```python
from build123d import *

# Parameters (mm, degrees)
SKETCH1_W                    = 52.8
SKETCH1_H                    = 30.6
EXT_BODY_DEPTH               = 13.8
AUTO_SWITCH_MOUNTING_DEPTH   = 57.677773421
SKETCH3_R                    = 8.5
CYL_BORE_DEPTH               = 2
M4X0_7_TAPPED_HOLE1_D        = 3.3
M4X0_7_TAPPED_HOLE1_DEPTH    = 10.1
M4X0_7_TAPPED_HOLE1_TIP      = 0.991420021
F_3_0_3_DIAMETER_HOLE1_D     = 3
F_3_0_3_DIAMETER_HOLE1_DEPTH = 3
F_3_0_3_DIAMETER_HOLE1_TIP   = 0.901290929
M4X0_7_TAPPED_HOLE2_D        = 3.3
M4X0_7_TAPPED_HOLE2_DEPTH    = 10.1
M4X0_7_TAPPED_HOLE2_TIP      = 0.991420021
M4X0_7_TAPPED_HOLE3_D        = 3.3
M4X0_7_TAPPED_HOLE3_DEPTH    = 10.1
M4X0_7_TAPPED_HOLE3_TIP      = 0.991420021
M4X0_7_TAPPED_HOLE4_D        = 3.3
M4X0_7_TAPPED_HOLE4_DEPTH    = 6.6
M4X0_7_TAPPED_HOLE4_TIP      = 0.991420021
M5X0_8_TAPPED_HOLE1_D        = 4.2
M5X0_8_TAPPED_HOLE1_DEPTH    = 6
M5X0_8_TAPPED_HOLE1_TIP      = 1.2618073
BOSS_EXTRUDE2_DEPTH          = 19
CHAMFER1_SIZE                = 0.25


with BuildPart() as part:
    # Sketch1 → EXT BODY (new, symmetric)
    with BuildSketch(Plane.XY):
        Rectangle(SKETCH1_W, SKETCH1_H)
    extrude(amount=EXT_BODY_DEPTH, both=True)

    # Sketch2 → AUTO SWITCH MOUNTING (cut, through all)
    with BuildSketch(Plane(origin=(26.4, 0, 0), x_dir=(0, 0, -1), z_dir=(1, 0, 0))):
        Polygon((2.5, 15.3), (-2.5, 15.3), (-2.5, 13.6), (-3.1, 13), (-3.1, 9.5), (3.1, 9.5), (3.1, 13), (2.5, 13.6), align=None)
        with BuildLine():
            Line((-13.022875656, 7.3), (-13.8, 7.3))
            Line((-13.8, 7.3), (-13.8, 4.3))
            Line((-13.8, 4.3), (-13.022875656, 4.3))
            ThreePointArc((-13.022875656, 4.3), (-9.7, 5.8), (-13.022875656, 7.3))
        make_face()
        with BuildLine():
            Line((-13.8, -7.3), (-13.8, -4.3))
            Line((-13.8, -4.3), (-13.022875656, -4.3))
            ThreePointArc((-13.022875656, -4.3), (-9.7, -5.8), (-13.022875656, -7.3))
            Line((-13.022875656, -7.3), (-13.8, -7.3))
        make_face()
        Polygon((-3.1, -9.5), (3.1, -9.5), (3.1, -13), (2.5, -13.6), (2.5, -15.3), (-2.5, -15.3), (-2.5, -13.6), (-3.1, -13), align=None)
        with BuildLine():
            Line((13.022875656, -7.3), (13.8, -7.3))
            Line((13.8, -7.3), (13.8, -4.3))
            Line((13.8, -4.3), (13.022875656, -4.3))
            ThreePointArc((13.022875656, -4.3), (9.7, -5.8), (13.022875656, -7.3))
        make_face()
        with BuildLine():
            Line((13.8, 7.3), (13.8, 4.3))
            Line((13.8, 4.3), (13.022875656, 4.3))
            ThreePointArc((13.022875656, 4.3), (9.7, 5.8), (13.022875656, 7.3))
            Line((13.022875656, 7.3), (13.8, 7.3))
        make_face()
    extrude(amount=-AUTO_SWITCH_MOUNTING_DEPTH, mode=Mode.SUBTRACT)

    # Sketch3 → CYL BORE (cut)
    with BuildSketch(Plane(origin=(26.4, 0, 0), x_dir=(0, 0, -1), z_dir=(1, 0, 0))):
        Circle(SKETCH3_R)
    extrude(amount=-CYL_BORE_DEPTH, mode=Mode.SUBTRACT)

    # M4x0.7 Tapped Hole1
    with Locations(Plane(origin=(26.4, 0, 0), x_dir=(0, 0, -1), z_dir=(1, 0, 0))):
        with Locations((-7.5, -11), (7.5, 11)):
            Hole(M4X0_7_TAPPED_HOLE1_D / 2, depth=M4X0_7_TAPPED_HOLE1_DEPTH)
            with Locations((0, 0, -(M4X0_7_TAPPED_HOLE1_DEPTH + M4X0_7_TAPPED_HOLE1_TIP / 2))):  # 118° drill point
                Cone(0, M4X0_7_TAPPED_HOLE1_D / 2, M4X0_7_TAPPED_HOLE1_TIP, mode=Mode.SUBTRACT)

    # Ø3.0 (3) Diameter Hole1
    with Locations(Plane(origin=(26.4, 0, 0), x_dir=(0, 0, -1), z_dir=(1, 0, 0))):
        with Locations((-6.5, 11)):
            Hole(F_3_0_3_DIAMETER_HOLE1_D / 2, depth=F_3_0_3_DIAMETER_HOLE1_DEPTH)
            with Locations((0, 0, -(F_3_0_3_DIAMETER_HOLE1_DEPTH + F_3_0_3_DIAMETER_HOLE1_TIP / 2))):  # 118° drill point
                Cone(0, F_3_0_3_DIAMETER_HOLE1_D / 2, F_3_0_3_DIAMETER_HOLE1_TIP, mode=Mode.SUBTRACT)

    # M4x0.7 Tapped Hole2
    with Locations(Plane.XY.offset(13.8)):
        with Locations((1.9, 12), (1.9, -12)):
            Hole(M4X0_7_TAPPED_HOLE2_D / 2, depth=M4X0_7_TAPPED_HOLE2_DEPTH)
            with Locations((0, 0, -(M4X0_7_TAPPED_HOLE2_DEPTH + M4X0_7_TAPPED_HOLE2_TIP / 2))):  # 118° drill point
                Cone(0, M4X0_7_TAPPED_HOLE2_D / 2, M4X0_7_TAPPED_HOLE2_TIP, mode=Mode.SUBTRACT)

    # M4x0.7 Tapped Hole3
    with Locations(Plane(origin=(0, 0, -13.8), x_dir=(-1, 0, 0), z_dir=(0, 0, -1))):
        with Locations((-1.9, 12), (-1.9, -12)):
            Hole(M4X0_7_TAPPED_HOLE3_D / 2, depth=M4X0_7_TAPPED_HOLE3_DEPTH)
            with Locations((0, 0, -(M4X0_7_TAPPED_HOLE3_DEPTH + M4X0_7_TAPPED_HOLE3_TIP / 2))):  # 118° drill point
                Cone(0, M4X0_7_TAPPED_HOLE3_D / 2, M4X0_7_TAPPED_HOLE3_TIP, mode=Mode.SUBTRACT)

    # M4x0.7 Tapped Hole4
    with Locations(Plane(origin=(0, 15.3, 0), x_dir=(1, 0, 0), z_dir=(0, 1, 0))):
        with Locations((-3.6, 8), (-3.6, -8)):
            Hole(M4X0_7_TAPPED_HOLE4_D / 2, depth=M4X0_7_TAPPED_HOLE4_DEPTH)
            with Locations((0, 0, -(M4X0_7_TAPPED_HOLE4_DEPTH + M4X0_7_TAPPED_HOLE4_TIP / 2))):  # 118° drill point
                Cone(0, M4X0_7_TAPPED_HOLE4_D / 2, M4X0_7_TAPPED_HOLE4_TIP, mode=Mode.SUBTRACT)

    # M5x0.8 Tapped Hole1
    with Locations(Plane(origin=(0, -15.3, 0), x_dir=(-1, 0, 0), z_dir=(0, -1, 0))):
        with Locations((-7.4, -7.5), (-18.9, 7.5)):
            Hole(M5X0_8_TAPPED_HOLE1_D / 2, depth=M5X0_8_TAPPED_HOLE1_DEPTH)
            with Locations((0, 0, -(M5X0_8_TAPPED_HOLE1_DEPTH + M5X0_8_TAPPED_HOLE1_TIP / 2))):  # 118° drill point
                Cone(0, M5X0_8_TAPPED_HOLE1_D / 2, M5X0_8_TAPPED_HOLE1_TIP, mode=Mode.SUBTRACT)

    # Sketch21 → Boss-Extrude2 (add, symmetric)
    with BuildSketch(Plane(origin=(0, 0, 0), x_dir=(1, 0, 0), z_dir=(0, 1, 0))):
        with BuildLine():
            Line((-33.9, 4.5), (-33.9, 11.25))
            Line((-33.9, 11.25), (-26.4, 11.25))
            Line((-26.4, 11.25), (-26.4, -11.25))
            Line((-26.4, -11.25), (-33.9, -11.25))
            Line((-33.9, -11.25), (-33.9, -4.5))
            Line((-33.9, -4.5), (-33.025, -4.5))
            ThreePointArc((-33.025, -4.5), (-32.025, -5.5), (-31.025, -4.5))
            Line((-31.025, -4.5), (-30.15, -4.5))
            Line((-30.15, -4.5), (-30.15, 4.5))
            Line((-30.15, 4.5), (-31.025, 4.5))
            ThreePointArc((-31.025, 4.5), (-32.025, 5.5), (-33.025, 4.5))
            Line((-33.025, 4.5), (-33.9, 4.5))
        make_face()
    extrude(amount=BOSS_EXTRUDE2_DEPTH, both=True)

    # Chamfer1
    chamfer1_edges = [part.edges().sort_by_distance(p)[0] for p in [
        (-33.9, 0, -4.5),
        (-33.9, 0, 4.5),
    ]]
    chamfer(chamfer1_edges, length=CHAMFER1_SIZE)


solid = part.part
```
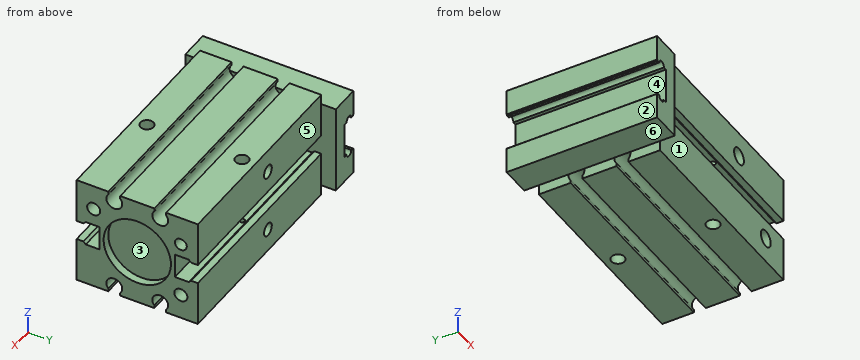
Geometry: final body of the model. Coordinates: model frame, mm. Face numbers are marked on the shaded views. A direction names the side the tool comes from. Round coordinates to 2 decimals unless told otherwise and drop trailing zeros. Write each loop counter-clockwise with the first axis right and the second up, starting at its lowest first coordinate (ties: lowest second). Pieces come first, ordered by that corner, then holes.
Item 1: Section query A-A (z = 0.25). Return loops of the section in (x, y), plus the area to 3 significant figures.
Item 2: Section query D-D (y = 5.5). Return loops of the section in (x, z) (3 decimals), plus the area to 3 significant figures.
Item 3: Mould query, pull axis Y, two halves, no side actions, for the marked faces 1, 2 and 3. Classes: +Y half, -Y half, draft (parallel to the pull), parting line (faces both ways), or undercut.
Item 4: Pin query (flat end, axial travel): P1, Ø0.5, axis at x = -33.5, y = 0.5, coming from the +Z side; P2, Ø12, axis at x = -12, z = 10.5, coming from the -Y side; P3, Ø3, axis at x = 1.9, y = -12, coming from the -Z side. Return the tip coordinate at first contact, or that it passes through.
Item 5: Set-up query: the marked faces 4, 5 and 6. Return all of +Z, -Z, +X, -X, +Y, -Y with unobstructed straight access to the full face (end or side cutting, diameter ignored); none if empty.
Item 6: Material intervals for L1, parallel to Y at x = -16, z = -11.7; L2, parallel to Y at x = 1.9, z = 8.5; L3, parallel to Z at x = 18.9, y = -13, sorted ascending.
Item 7: Section query C-C (x = 1.9). Give the number of separate pieces and of enclosed holes in the cut face, plus the area to 3 significant figures.
Item 8: Section query B-B (y = -5.8). Return loops of the section in (x, z) (3 decimals).
Completed:
1. outline: (-30.15, -19) - (-26.4, -19) - (-26.4, -9.5) - (26.4, -9.5) - (26.4, -8.5) - (24.4, -8.5) - (24.4, 8.5) - (26.4, 8.5) - (26.4, 9.5) - (-26.4, 9.5) - (-26.4, 19) - (-30.15, 19) - close
1. area: 1,110 mm2
2. outline: (-33.9, -11.25) - (-26.4, -11.25) - (-26.4, -9.723) - (26.4, -9.723) - (26.4, -6.481) - (24.4, -6.481) - (24.4, 6.481) - (26.4, 6.481) - (26.4, 9.723) - (-26.4, 9.723) - (-26.4, 11.25) - (-33.9, 11.25) - (-33.9, 4.75) - (-33.65, 4.5) - (-33.025, 4.5) arc R1 cw to (-31.025, 4.5) - (-30.15, 4.5) - (-30.15, -4.5) - (-31.025, -4.5) arc R1 cw to (-33.025, -4.5) - (-33.65, -4.5) - (-33.9, -4.75) - close
2. area: 1,130 mm2
3. face 1: -Y half
3. face 2: draft
3. face 3: undercut
4. P1: stops at z = 11.25
4. P2: stops at y = -15.3
4. P3: stops at z = -3.61
5. face 4: -X, +Y, -Y
5. face 5: +Z, -Z, +X, +Y
5. face 6: -Z, -X, +Y, -Y
6. L1: y = -15.3 to -7.8, -3.8 to 3.8, 7.8 to 15.3
6. L2: y = -15.3 to -13.65, -10.35 to 10.35, 13.65 to 15.3
6. L3: z = -13.8 to -9.6, -5.4 to -3.1, 3.1 to 13.8
7. separate pieces: 5
7. enclosed holes: 0
7. area: 585 mm2
8. outline: (-33.9, -11.25) - (-26.4, -11.25) - (-26.4, -9.7) - (26.4, -9.7) - (26.4, -6.214) - (24.4, -6.214) - (24.4, 6.214) - (26.4, 6.214) - (26.4, 9.7) - (-26.4, 9.7) - (-26.4, 11.25) - (-33.9, 11.25) - (-33.9, 4.75) - (-33.65, 4.5) - (-33.025, 4.5) arc R1 cw to (-31.025, 4.5) - (-30.15, 4.5) - (-30.15, -4.5) - (-31.025, -4.5) arc R1 cw to (-33.025, -4.5) - (-33.65, -4.5) - (-33.9, -4.75) - close
